```python
from build123d import *

# Parameters (mm, degrees)
F0_W     = 145
F0_H     = 54
F1_DEPTH = 200


with BuildPart() as f1:
    # F0 (on Right) → F1 (new body)
    with BuildSketch(Plane.YZ):
        with Locations((72.5, 27)):
            Rectangle(F0_W, F0_H)
        with BuildLine():
            Line((69, 50.2), (72.5, 50.2))
            Line((72.5, 50.2), (76, 50.2))
            Line((76, 50.2), (76, 51.5))
            Line((76, 51.5), (103, 51.5))
            Line((103, 51.5), (103, 50.2))
            Line((103, 50.2), (110, 50.2))
            Line((110, 50.2), (110, 51.5))
            Line((110, 51.5), (128, 51.5))
            Line((128, 51.5), (128, 50.2))
            Line((128, 50.2), (136.45, 50.2))
            Line((136.45, 50.2), (136.45, 49.6))
            ThreePointArc((136.45, 49.6), (137.6, 48.45), (138.75, 49.6))
            ThreePointArc((138.75, 49.6), (141.737437, 50.837437), (140.5, 47.85))
            ThreePointArc((140.5, 47.85), (139.35, 46.7), (140.5, 45.55))
            Line((140.5, 45.55), (142.6, 45.55))
            Line((142.6, 45.55), (142.6, 43.5))
            Line((142.6, 43.5), (140, 43.5))
            Line((140, 43.5), (140, 41.9))
            Line((140, 41.9), (142.6, 41.9))
            Line((142.6, 41.9), (142.6, 36.1))
            Line((142.6, 36.1), (140, 36.1))
            Line((140, 36.1), (140, 34.5))
            Line((140, 34.5), (142.6, 34.5))
            Line((142.6, 34.5), (142.6, 32.682376))
            Line((142.6, 32.682376), (140, 32.682376))
            Line((140, 32.682376), (140.9, 27))
            Line((140.9, 27), (140, 21.317624))
            Line((140, 21.317624), (142.6, 21.317624))
            Line((142.6, 21.317624), (142.6, 19.5))
            Line((142.6, 19.5), (140, 19.5))
            Line((140, 19.5), (140, 17.9))
            Line((140, 17.9), (142.6, 17.9))
            Line((142.6, 17.9), (142.6, 12.1))
            Line((142.6, 12.1), (140, 12.1))
            Line((140, 12.1), (140, 10.5))
            Line((140, 10.5), (142.6, 10.5))
            Line((142.6, 10.5), (142.6, 8.45))
            Line((142.6, 8.45), (140.5, 8.45))
            ThreePointArc((140.5, 8.45), (139.35, 7.3), (140.5, 6.15))
            ThreePointArc((140.5, 6.15), (141.737437, 3.162563), (138.75, 4.4))
            ThreePointArc((138.75, 4.4), (137.6, 5.55), (136.45, 4.4))
            Line((136.45, 4.4), (136.45, 3.8))
            Line((136.45, 3.8), (128, 3.8))
            Line((128, 3.8), (128, 2.5))
            Line((128, 2.5), (110, 2.5))
            Line((110, 2.5), (110, 3.8))
            Line((110, 3.8), (103, 3.8))
            Line((103, 3.8), (103, 2.5))
            Line((103, 2.5), (76, 2.5))
            Line((76, 2.5), (76, 3.8))
            Line((76, 3.8), (72.5, 3.8))
            Line((72.5, 3.8), (69, 3.8))
            Line((69, 3.8), (69, 2.5))
            Line((69, 2.5), (42, 2.5))
            Line((42, 2.5), (42, 3.8))
            Line((42, 3.8), (35, 3.8))
            Line((35, 3.8), (35, 2.5))
            Line((35, 2.5), (17, 2.5))
            Line((17, 2.5), (17, 3.8))
            Line((17, 3.8), (8.55, 3.8))
            Line((8.55, 3.8), (8.55, 4.4))
            ThreePointArc((8.55, 4.4), (7.4, 5.55), (6.25, 4.4))
            ThreePointArc((6.25, 4.4), (3.262563, 3.162563), (4.5, 6.15))
            ThreePointArc((4.5, 6.15), (5.65, 7.3), (4.5, 8.45))
            Line((4.5, 8.45), (2.4, 8.45))
            Line((2.4, 8.45), (2.4, 10.5))
            Line((2.4, 10.5), (5, 10.5))
            Line((5, 10.5), (5, 12.1))
            Line((5, 12.1), (2.4, 12.1))
            Line((2.4, 12.1), (2.4, 17.9))
            Line((2.4, 17.9), (5, 17.9))
            Line((5, 17.9), (5, 19.5))
            Line((5, 19.5), (2.4, 19.5))
            Line((2.4, 19.5), (2.4, 21.317624))
            Line((2.4, 21.317624), (5, 21.317624))
            Line((5, 21.317624), (4.1, 27))
            Line((4.1, 27), (5, 32.682376))
            Line((5, 32.682376), (2.4, 32.682376))
            Line((2.4, 32.682376), (2.4, 34.5))
            Line((2.4, 34.5), (5, 34.5))
            Line((5, 34.5), (5, 36.1))
            Line((5, 36.1), (2.4, 36.1))
            Line((2.4, 36.1), (2.4, 41.9))
            Line((2.4, 41.9), (5, 41.9))
            Line((5, 41.9), (5, 43.5))
            Line((5, 43.5), (2.4, 43.5))
            Line((2.4, 43.5), (2.4, 45.55))
            Line((2.4, 45.55), (4.5, 45.55))
            ThreePointArc((4.5, 45.55), (5.65, 46.7), (4.5, 47.85))
            ThreePointArc((4.5, 47.85), (3.262563, 50.837437), (6.25, 49.6))
            ThreePointArc((6.25, 49.6), (7.4, 48.45), (8.55, 49.6))
            Line((8.55, 49.6), (8.55, 50.2))
            Line((8.55, 50.2), (17, 50.2))
            Line((17, 50.2), (17, 51.5))
            Line((17, 51.5), (35, 51.5))
            Line((35, 51.5), (35, 50.2))
            Line((35, 50.2), (42, 50.2))
            Line((42, 50.2), (42, 51.5))
            Line((42, 51.5), (69, 51.5))
            Line((69, 51.5), (69, 50.2))
        make_face(mode=Mode.SUBTRACT)
    extrude(amount=F1_DEPTH)


solid = f1.part
```
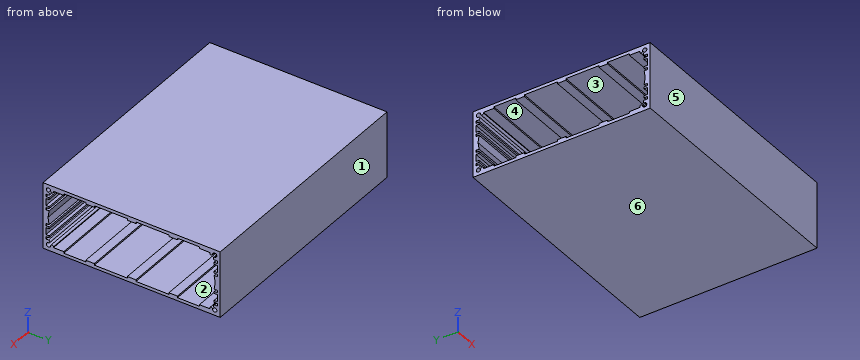
Read the model definition and answer for the solid it produces. Units are mm, in the model's axes. Face numbers are marked on the shaded views. A direction names the side the tool comes from. Coordinates: 2 decimals unless noted, no trailing zeros. Loops run counter-clockwise (first coordinate to the right, second up) from the corner with the lowest first, then second, coordinate; pieces in that order, holes last.
(1) Consider line 1 along Y through (x, z) = (107.5, 4.4); line 2 along Z through (x, y) = (164, 99.5). Determine where each line is inside the solid, lowest interval first.
Solution:
line 1: y = 0 to 2.75, 6.25 to 8.55, 136.45 to 138.75, 142.25 to 145
line 2: z = 0 to 2.5, 51.5 to 54
(2) The mould has two halves that part along Z. Classify the marked faces 3, 4, 5 and 6: released by +Z, released by -Z, zero draft, split by the parting line, or undercut.
Solution:
face 3: undercut
face 4: undercut
face 5: zero draft
face 6: released by -Z
(3) A flat-ended cylindrical pin translates along its axis: pin 1 Ø3 at (y, z) = (140.5, 4.4) entering from -X. Find the tip coordinate at first contact, or state that the pin passes through.
Solution:
pin 1: passes through
(4) A tool of negligible diameter and unlimited length cuts with its end or side. For the marked faces 1 and 2, from which of +Z, -Z, +X, -X, +Y, -Y can it reach the whole face along a straight path? Write none if from no direction.
Solution:
face 1: +Z, -Z, +X, -X, +Y
face 2: +X, -X
(5) The part is cut by section A-A (y = 50). Determine the outline of the cut face in (x, z).
Solution:
outline: (0, 0) - (200, 0) - (200, 2.5) - (0, 2.5) - close; (0, 51.5) - (200, 51.5) - (200, 54) - (0, 54) - close
